The listing builds one solid part. Answer for the finished solid, in the listing's coordinates (mm). A direction names the side the tool comes from. Coordinates: 2 decimals unless noted, no trailing zeros. Order: outer loops, then holes, each group sorted by start corner. A loop starts at its lowest first (then second) coordinate and runs counter-clockwise, first axis right, second up. Notation, with made-up numbers: (62.5, -36.75) - (110.5, -36.75) arc R27 cw to (110.5, -15.75) - close; hole circle Ø4 at (41, -9). An arc over 180 degrees is marked (long way). Use one line per item in the form item = value. Start each with the question number.
Item 1: Each of these flat-tipped pins is pushed along its axis until it touches: pin 1 Ø1 at (y, z) = (6.5, 3.5) entering from +X; pin 2 Ø3 at (y, z) = (17.5, 2) entering from +X; pin 3 Ø6.5 at (y, z) = (-30, 10) entering from -X. Where does it stop, or does it pass through?
Item 2: A tool of negligible diameter and unlimited length cuts with its end or side. For faces 1 (the cylindrical face through (74.826, -16.429, 9.902)), 2 (the flat face through (18, 0, 0)), 3 (the flat face through (-120.5, 0, 11)), 4 (the flat face through (-56.5, 0, 2)), 5 (the flat face through (-53.5, -28, 10)), from which of +Z, -Z, +X, -X, +Y, -Y can it reach the whole face along a straight path? Write none if from no direction.
Item 3: Consider line 1 along Y through (x, z) = (37, 12.25); line 2 along Y through (x, z) = (96, 8.5); line 3 along X through (y, z) = (-3, 8.5). Determine where each line is inside the solid, lowest interval first. Write a range as [from, to].
Item 4: The mould has two halves that part along X. Classify faces 6 (the flat face through (-53.5, 28, 10)), 7 (the flat face through (-89, -15.5, 11)), 8 (the cylindrical face through (133.743, 0.825, 9.902)), 9 (the flat face through (-88, 18.5, 11)): released by +X, released by -X, zero draft, split by the parting line, or undercut.
Item 5: Section A-A, the plane y = 0 is taken. Write down the section's boundary in (x, z).
Item 6: Section B-B, the plane x = 29.5 is taken. Write down the section's boundary in (y, z), and give its area (3 significant figures).
from build123d import *

# Parameters (mm, degrees)
BOSS_EXTRUDE1_DEPTH = 17
FILLET1_R           = 3
SHELL2_START        = 3
SHELL2_DEPTH        = 14
CUT_EXTRUDE1_START  = 3
SKETCH2_W           = 3
SKETCH2_H           = 69.184745233
CUT_EXTRUDE1_DEPTH  = 14
SKETCH4_R           = 24
BOSS_EXTRUDE2_DEPTH = 17
SHELL4_START        = 3
SHELL4_OUTLINE_R    = 27
SHELL4_DEPTH        = 14
SKETCH7_W           = 3
SKETCH7_H           = 69
CUT_EXTRUDE3_DEPTH  = 14
SKETCH8_R           = 3.051675087
CUT_EXTRUDE4_DEPTH  = 20
SKETCH9_R           = 3.853535646
SKETCH9_R_2         = 3.770722203
CUT_EXTRUDE5_DEPTH  = 20
SKETCH11_W          = 68.674120891
SKETCH11_H          = 38.021066824
CUT_EXTRUDE8_DEPTH  = 5
SKETCH15_W          = 10
SKETCH15_H          = 2
BOSS_EXTRUDE3_DEPTH = 1
CHAMFER1_SIZE       = 1
SKETCH14_W          = 10
SKETCH14_H          = 2
BOSS_EXTRUDE4_DEPTH = 1
CHAMFER2_SIZE       = 1
FILLET2_R           = 3
SKETCH16_R          = 3.2
CUT_EXTRUDE9_DEPTH  = 3


# Read off the part's stored shape, not the designer's step: Shell2, Shell4
with BuildPart() as part:
    # Sketch1 → Boss-Extrude1 (new body)
    with BuildSketch(Plane.XY):
        Polygon((-53.5, -18.5), (-53.5, -37.5), (53.5, -37.5), (53.5, 37.5), (-53.5, 37.5), (-53.5, 18.5), (-123.5, 18.5), (-123.5, -18.5), align=None)
    extrude(amount=BOSS_EXTRUDE1_DEPTH)

    # Fillet1
    fillet1_edges = [part.edges().sort_by_distance(p)[0] for p in [
        (-53.5, -37.5, 8.5),
        (-53.5, -18.5, 8.5),
        (-123.5, -18.5, 8.5),
        (-123.5, 18.5, 8.5),
        (-53.5, 18.5, 8.5),
        (-53.5, 37.5, 8.5),
    ]]
    fillet(fillet1_edges, radius=FILLET1_R)

    # Shell2 outline → Shell2 (cut)
    with BuildSketch(Plane.XY.offset(SHELL2_START)):
        with BuildLine():
            Line((50.5, -34.5), (50.5, 34.5))
            Line((50.5, 34.5), (-50.5, 34.5))
            Line((-50.5, 34.5), (-50.5, 21.5))
            ThreePointArc((-50.5, 21.5), (-52.257359313, 17.257359313), (-56.5, 15.5))
            Line((-56.5, 15.5), (-120.5, 15.5))
            Line((-120.5, 15.5), (-120.5, -15.5))
            Line((-120.5, -15.5), (-56.5, -15.5))
            ThreePointArc((-56.5, -15.5), (-52.257359313, -17.257359313), (-50.5, -21.5))
            Line((-50.5, -21.5), (-50.5, -34.5))
            Line((-50.5, -34.5), (50.5, -34.5))
        make_face()
    extrude(amount=SHELL2_DEPTH, mode=Mode.SUBTRACT)

    # Sketch2 → Cut-Extrude1 (cut)
    with BuildSketch(Plane.XY.offset(CUT_EXTRUDE1_START)):
        with Locations((52, -0.092372617)):
            Rectangle(SKETCH2_W, SKETCH2_H)
    extrude(amount=CUT_EXTRUDE1_DEPTH, mode=Mode.SUBTRACT)

    # Sketch4 → Boss-Extrude2 (add)
    with BuildSketch(Plane.XY):
        with BuildLine():
            Line((53.5, 37.5), (96.25236473, 37.5))
            ThreePointArc((96.25236473, 37.5), (133.75236473, 0), (96.25236473, -37.5))
            Line((96.25236473, -37.5), (53.5, -37.5))
            Line((53.5, -37.5), (53.5, 37.5))
        make_face()
        with Locations((96.25236473, 0)):
            Circle(SKETCH4_R, mode=Mode.SUBTRACT)
    extrude(amount=BOSS_EXTRUDE2_DEPTH)

    # Shell4 outline → Shell4 (cut)
    with BuildSketch(Plane.XY.offset(SHELL4_START)):
        with BuildLine():
            Line((96.25236473, 34.5), (56.5, 34.5))
            Line((56.5, 34.5), (56.5, -34.5))
            Line((56.5, -34.5), (96.25236473, -34.5))
            ThreePointArc((96.25236473, -34.5), (130.75236473, 0), (96.25236473, 34.5))
        make_face()
        with Locations((96.25236473, 0)):
            Circle(SHELL4_OUTLINE_R, mode=Mode.SUBTRACT)
    extrude(amount=SHELL4_DEPTH, mode=Mode.SUBTRACT)

    # Sketch7 → Cut-Extrude3 (cut)
    with BuildSketch(Plane.XY.offset(17)):
        with Locations((55, 0)):
            Rectangle(SKETCH7_W, SKETCH7_H)
    extrude(amount=-CUT_EXTRUDE3_DEPTH, mode=Mode.SUBTRACT)

    # Sketch8 → Cut-Extrude4 (cut)
    with BuildSketch(Plane(origin=(0, 0, 0), x_dir=(-1, 0, 0), z_dir=(0, 0, -1))):
        with Locations((47.431025643, -31.425786946)):
            Circle(SKETCH8_R)
        with Locations((47.407650962, 31.49020456)):
            Circle(SKETCH8_R)
        with Locations((-61.783104826, 31.350542021)):
            Circle(SKETCH8_R)
        with Locations((-61.783104826, -31.425786946)):
            Circle(SKETCH8_R)
    extrude(amount=-CUT_EXTRUDE4_DEPTH, mode=Mode.SUBTRACT)

    # Sketch9 → Cut-Extrude5 (cut)
    with BuildSketch(Plane(origin=(0, 37.5, 0), x_dir=(1, 0, 0), z_dir=(0, 1, 0))):
        with Locations((-30.827052477, -17)):
            Circle(SKETCH9_R)
        with Locations((-10.906615981, -16.992280087)):
            Circle(SKETCH9_R_2)
    extrude(amount=-CUT_EXTRUDE5_DEPTH, mode=Mode.SUBTRACT)

    # Sketch11 → Cut-Extrude8 (cut)
    with BuildSketch(Plane(origin=(0, 0, 0), x_dir=(-1, 0, 0), z_dir=(0, 0, -1))):
        with Locations((90.837060446, -0.510533412)):
            Rectangle(SKETCH11_W, SKETCH11_H)
    extrude(amount=-CUT_EXTRUDE8_DEPTH, mode=Mode.SUBTRACT)

    # Sketch15 → Boss-Extrude3 (add)
    with BuildSketch(Plane.XZ.offset(-15.5)):
        with Locations((-71.5, 8)):
            Rectangle(SKETCH15_W, SKETCH15_H)
        with Locations((-105.5, 8)):
            Rectangle(SKETCH15_W, SKETCH15_H)
    extrude(amount=BOSS_EXTRUDE3_DEPTH)

    # Chamfer1
    chamfer1_edges = [part.edges().sort_by_distance(p)[0] for p in [
        (-105.5, 14.5, 9),
        (-105.5, 14.5, 7),
        (-71.5, 14.5, 9),
        (-71.5, 14.5, 7),
    ]]
    chamfer(chamfer1_edges, length=CHAMFER1_SIZE - 0.0001)  # a hair under: the kernel refuses the full size

    # Sketch14 → Boss-Extrude4 (add)
    with BuildSketch(Plane(origin=(0, -15.5, 0), x_dir=(1, 0, 0), z_dir=(0, 1, 0))):
        with Locations((-71.5, -8)):
            Rectangle(SKETCH14_W, SKETCH14_H)
        with Locations((-105.5, -8)):
            Rectangle(SKETCH14_W, SKETCH14_H)
    extrude(amount=BOSS_EXTRUDE4_DEPTH)

    # Chamfer2
    chamfer2_edges = [part.edges().sort_by_distance(p)[0] for p in [
        (-105.5, -14.5, 7),
        (-105.5, -14.5, 9),
        (-71.5, -14.5, 9),
        (-71.5, -14.5, 7),
    ]]
    chamfer(chamfer2_edges, length=CHAMFER2_SIZE - 0.0001)  # a hair under: the kernel refuses the full size

    # Fillet2
    fillet2_edges = [part.edges().sort_by_distance(p)[0] for p in [
        (72.25236473, 0, 0),
        (133.75236473, 0, 0),
        (22.876182365, 37.5, 0),
        (22.876182365, -37.5, 0),
        (-53.5, -28, 0),
        (-53.5, 28, 0),
        (-52.621320344, 36.621320344, 0),
        (-52.621320344, -36.621320344, 0),
        (-54.378679656, -19.378679656, 0),
        (-54.378679656, 19.378679656, 0),
    ]]
    fillet(fillet2_edges, radius=FILLET2_R)

    # Sketch16 → Cut-Extrude9 (cut)
    with BuildSketch(Plane(origin=(0, 0, 0), x_dir=(-1, 0, 0), z_dir=(0, 0, -1))):
        with Locations((38.150596078, -9.60262109)):
            Circle(SKETCH16_R)
    extrude(amount=-CUT_EXTRUDE9_DEPTH, mode=Mode.SUBTRACT)


solid = part.part
Response:
q1.pin_1 = 133.27
q1.pin_2 = 130.08
q1.pin_3 = -53.5
q2.face_1 = +Z
q2.face_2 = -Z, +X, -X, +Y, -Y
q2.face_3 = +Z, -Z
q2.face_4 = -Z, -X, +Y, -Y
q2.face_5 = +Z, -Z, -X, -Y
q3.line_1 = [-37.5, -34.5], [34.5, 37.5]
q3.line_2 = [-37.5, -34.5], [-27, -24], [24, 27], [34.5, 37.5]
q3.line_3 = [-123.5, -120.5], [69.42, 72.44], [120.06, 123.09], [130.62, 133.63]
q4.face_6 = released by -X
q4.face_7 = undercut
q4.face_8 = released by +X
q4.face_9 = zero draft
q5.outline = (-123.5, 5) - (-120.5, 5) - (-120.5, 17) - (-123.5, 17) - close; (-56.5, 0) - (69.25, 0) arc R3 ccw to (72.25, 3) - (72.25, 17) - (69.25, 17) - (69.25, 3) - (-56.5, 3) - close; (120.25, 3) arc R3 ccw to (123.25, 0) - (130.75, 0) arc R3 ccw to (133.75, 3) - (133.75, 17) - (130.75, 17) - (130.75, 3) - (123.25, 3) - (123.25, 17) - (120.25, 17) - close
q6.outline = (-37.5, 3) arc R3 ccw to (-34.5, 0) - (34.5, 0) arc R3 ccw to (37.5, 3) - (37.5, 17) - (34.5, 17) - (34.5, 3) - (-34.5, 3) - (-34.5, 17) - (-37.5, 17) - close
q6.area = 305 mm2
